```python
from build123d import *

# Parameters (mm, degrees)
BOSS_EXTRUDE1_DEPTH = 5
SKETCH2_R           = 3
BOSS_EXTRUDE2_DEPTH = 10
SKETCH3_R           = 1.5
CUT_EXTRUDE1_DEPTH  = 19.953891421


with BuildPart() as part:
    # Sketch1 → Boss-Extrude1 (new body)
    with BuildSketch(Plane.XY):
        with BuildLine():
            Line((0, -12.5), (0, 12.5))
            ThreePointArc((0, 12.5), (0.585786438, 13.914213562), (2, 14.5))
            Line((2, 14.5), (5, 14.5))
            ThreePointArc((5, 14.5), (6.414213562, 13.914213562), (7, 12.5))
            Line((7, 12.5), (7, -12.5))
            ThreePointArc((7, -12.5), (6.414213562, -13.914213562), (5, -14.5))
            Line((5, -14.5), (2, -14.5))
            ThreePointArc((2, -14.5), (0.585786438, -13.914213562), (0, -12.5))
        make_face()
    extrude(amount=BOSS_EXTRUDE1_DEPTH)

    # Sketch2 → Boss-Extrude2 (add)
    with BuildSketch(Plane.XY.offset(5)):
        with Locations((3.5, 0)):
            Circle(SKETCH2_R)
    extrude(amount=BOSS_EXTRUDE2_DEPTH)

    # Sketch3 → Cut-Extrude1 (cut, through all)
    with BuildSketch(Plane.XY.offset(5)):
        with Locations((3.5, 8)):
            Circle(SKETCH3_R)
        with Locations((3.5, -8)):
            Circle(SKETCH3_R)
    extrude(amount=-CUT_EXTRUDE1_DEPTH, mode=Mode.SUBTRACT)


solid = part.part
```
Model file for the job. Use its own axes, mm. A direction names the side the tool comes from. Coordinates: 2 decimals unless noted, no trailing zeros. Order: outer loops, then holes, each group sorted by start corner. A loop starts at its lowest first (then second) coordinate and runs counter-clockwise, first axis right, second up. Notation, with made-up numbers: (42.25, 77.25) - (51.25, 77.25) arc R24 cw to (51.25, 107.25) - close; hole circle Ø7 at (-21, -1). An arc over 180 degrees is marked (long way). Return JSON: item names as keys, results as strings. Group by question number.
1) Flat gauge pins, fed straight in: P1, Ø2, axis at x = 5, y = 5.5, coming from the +Z side; P2, Ø8, axis at y = 0, z = 12.5, coming from the -X side; P3, Ø1, axis at x = 1, z = 3, coming from the -Y side. Where does each tip first touch, or does it go through?
2) Mould opens along Y. For faces 3 (the cylindrical face through (0.57, 13.9, 2.46)), 4 (the cylindrical face through (4.19, 6.67, 2.54)), 5 (the flat face through (0, 0, 2)) say: released by +Y, released by -Y, zero draft, split by the parting line, or undercut.
3) Tool access for faces 1 (the cylindrical face through (4.19, -9.33, 2.54)), 2 (the cylindrical face through (0.5, 0.1, 9.9)): list every direction of +Z, -Z, +X, -X, +Y, -Y with a clear straight run to the whole face (end or side of a thin tool).
4) Saw through at B-B, the plane x = 3.5. Write the cut outline in (y, z), plus the area to 3 significant figures.
5) Probe line 1 (Y direction, x = 3.5, z = 1.7); line 2 (Z direction, x = 1, y = 6.75); line 3 (Y direction, x = 5.5, z = 13.75). List the from-to ranges inside material, lowest first. Write a range as from..to.
6) Saw through at C-C, the plane y = 0. Write the cut outline in (x, z), plus the area to 3 significant figures.
7) Saw through at D-D, the plane z = 14. Write the cut outline in (x, y).
8) Saw through at A-A, the plane y = 8. Write the cut outline in (x, z), plus the area to 3 significant figures.
Values found:
{
 "1": {"P1": "stops at z = 5", "P2": "stops at x = 0.5", "P3": "stops at y = -14.44"},
 "2": {"face 3": "released by +Y", "face 4": "undercut", "face 5": "zero draft"},
 "3": {"face 1": "+Z, -Z", "face 2": "+Z"},
 "4": {"outline": "(-14.5, 0) - (-9.5, 0) - (-9.5, 5) - (-14.5, 5) - close; (-6.5, 0) - (6.5, 0) - (6.5, 5) - (3, 5) - (3, 15) - (-3, 15) - (-3, 5) - (-6.5, 5) - close; (9.5, 0) - (14.5, 0) - (14.5, 5) - (9.5, 5) - close", "area": "175 mm²"},
 "5": {"line 1": "y = -14.5..-9.5, -6.5..6.5, 9.5..14.5", "line 2": "z = 0..5", "line 3": "y = -2.24..2.24"},
 "6": {"outline": "(0, 0) - (7, 0) - (7, 5) - (6.5, 5) - (6.5, 15) - (0.5, 15) - (0.5, 5) - (0, 5) - close", "area": "95.0 mm²"},
 "7": {"outline": "circle Ø6 at (3.5, 0)"},
 "8": {"outline": "(0, 0) - (2, 0) - (2, 5) - (0, 5) - close; (5, 0) - (7, 0) - (7, 5) - (5, 5) - close", "area": "20.0 mm²"}
}
